For this review, take the finished solid that the model builds, in its own axes (mm). A direction names the side the tool comes from. Give positions to 0.01 mm unless a question says otherwise; leave off trailing zeros. Write each loop counter-clockwise with the first axis right and the second up, starting at its lowest first coordinate (ties: lowest second). Pieces come first, ordered by that corner, then holes. Notation, with made-up numbers: M 77,-4 L 135,-4 A27 cw 135,26 Z; hole C 47,-28.5 d7. An arc over 180 degrees is marked long. One line per item, written item: value. Start each with the question number.
Item 1: To check wall thickness, follow probe 1 along X at (y, z) = (-0.9, 15); probe 2 along X at (y, z) = (2.5, 4); probe 3 along X at (y, z) = (-1.5, 21.25). State the ranges of each line that lie inside material, in increasing order.
Item 2: Consider section D-D, the plane z = 15. Write out the cut boundary in (x, y), and give its area (3 significant figures).
Item 3: Tool access review of faces 1 (the face through (31.879, 2.186, 14.79)), 2 (the face through (38.4, 1.2, 14.8)): name each direction out of +Z, -Z, +X, -X, +Y, -Y from which nothing blocks a thin tool from reaching the whole face with its end or side.
Item 4: Consider section B-B, the plane x = 0. Write out the cut boundary in (y, z).
Item 5: Clearance check with flat-ended pins moving along their axes: pin 1 Ø1.2 at (y, z) = (-1, 17.5) entering from -X; pin 2 Ø1.2 at (y, z) = (-1.5, 11.5) entering from +X; pin 3 Ø9 at (x, z) = (13, 17.5) entering from +Y. State where each tip first meets the part, or that it passes through.
Item 6: Consider section A-A, the plane z = 12. Write out the cut boundary in (x, y), and give its area (3 significant figures).
Item 7: Mouldability with a two-part tool opening along X and no side actions: class faces 3 (the face through (0, 2.071, 8)), 4 (the face through (-38.4, 1.2, 14.8)), 5 (the face through (-1, 0, 0)) as released by +X, released by -X, zero draft, split by the parting line, or undercut.
Item 8: Consider section C-C, the plane z = 5.5. Write out the cut boundary in (x, y).
```python
from build123d import *

# Parameters (mm, degrees)
BOSS_EXTRUDE1_DEPTH = 30
FILLET1_R           = 5
SKETCH2_R           = 5
CUT_EXTRUDE1_DEPTH  = 30


with BuildPart() as part:
    # Sketch1 → Boss-Extrude1 (new body)
    with BuildSketch(Plane.XY):
        Polygon((37.92, -2.070510622), (37.92, 2.070510622), (35.334085277, 2.070510622), (33.1622407, 1.057762863), (33.014324308, 1.374970589), (34.505914723, 2.070510622), (31.92, 2.070510622), (-31.92, 2.070510622), (-34.505914723, 2.070510622), (-33.014324308, 1.374970589), (-33.1622407, 1.057762863), (-35.334085277, 2.070510622), (-37.92, 2.070510622), (-37.92, -2.070510622), align=None)
        Polygon((-39.732615574, 2.915747145), (-37.92, 2.070510622), (-35.334085277, 2.070510622), (-39.270755184, 3.906209947), align=None)
        Polygon((-34.505914723, 2.070510622), (-31.92, 2.070510622), (-38.660978403, 5.213880475), (-39.122838793, 4.223417673), align=None)
        Polygon((31.92, 2.070510622), (34.505914723, 2.070510622), (39.122838793, 4.223417673), (38.660978403, 5.213880475), align=None)
        Polygon((35.334085277, 2.070510622), (37.92, 2.070510622), (39.732615574, 2.915747145), (39.270755184, 3.906209947), align=None)
    extrude(amount=BOSS_EXTRUDE1_DEPTH)

    # Fillet1
    # the kernel refuses this fillet: 5 mm, written as the material it adds along each edge
    with BuildSketch(Plane(origin=(37.92, 2.070510622, 0), x_dir=(0, -1, 0), z_dir=(0, 0, 1))) as fillet1_piece_1:
        with BuildLine():
            CenterArc((3.007110881, 5), FILLET1_R, 219.603933445, 50.396066555)
            Line((-0.845236523, 1.812615574), (-0.922283472, 1.748867886))
            ThreePointArc((-0.922283472, 1.748867886), (-0.51324904, 0.864045961), (-0.090630779, -0.042261826))
            Line((-0.090630779, -0.042261826), (0, -0.1))
            Line((0, -0.1), (3.007110881, -0.1))
            Line((3.007110881, -0.1), (3.007110881, 0))
        make_face()
    extrude(amount=30)
    with BuildSketch(Plane(origin=(-37.92, 2.070510622, 0), x_dir=(0, -1, 0), z_dir=(0, 0, 1))) as fillet1_piece_2:
        with BuildLine():
            CenterArc((3.007110881, -5), FILLET1_R, 90, 50.396066555)
            Line((-0.845236523, -1.812615574), (-0.922283472, -1.748867886))
            ThreePointArc((-0.922283472, -1.748867886), (-0.51324904, -0.864045961), (-0.090630779, 0.042261826))
            Line((-0.090630779, 0.042261826), (0, 0.1))
            Line((0, 0.1), (3.007110881, 0.1))
            Line((3.007110881, 0.1), (3.007110881, 0))
        make_face()
    extrude(amount=30)
    with BuildSketch(Plane(origin=(31.92, 2.070510622, 0), x_dir=(-1, 0, 0), z_dir=(0, 0, 1)), Plane(origin=(-31.92, 2.070510622, 0), x_dir=(-0.9063077870366495, 0.4226182617407004, 0), z_dir=(0, 0, 1))) as fillet1_piece_3:
        with BuildLine():
            CenterArc((FILLET1_R * 0.221694662643, -FILLET1_R), FILLET1_R, 90, 25)
            Line((-FILLET1_R * 0.200923599098, -FILLET1_R * 0.0936922129634), (-FILLET1_R * 0.209375964333, -FILLET1_R * 0.0755660572226))
            Line((-FILLET1_R * 0.209375964333, -FILLET1_R * 0.0755660572226), (-FILLET1_R * 0.00443389325286, FILLET1_R * 0.02))
            Line((-FILLET1_R * 0.00443389325286, FILLET1_R * 0.02), (FILLET1_R * 0.221694662643, FILLET1_R * 0.02))
            Line((FILLET1_R * 0.221694662643, FILLET1_R * 0.02), (FILLET1_R * 0.221694662643, 0))
        make_face()
    extrude(amount=30)

    # Sketch2 → Cut-Extrude1 (cut)
    with BuildSketch(Plane(origin=(0, 2.070510622, 0), x_dir=(1, 0, 0), z_dir=(0, 1, 0))):
        with Locations(Location((0, -15, 0), (0, 0, 270))):
            Circle(SKETCH2_R)
    extrude(amount=-CUT_EXTRUDE1_DEPTH, mode=Mode.SUBTRACT)


solid = part.part
```
Model answer:
1. probe 1: x = -37.92 to -5, 5 to 37.92
1. probe 2: x = -39.29 to -36.26, -35.43 to -32.84, 32.84 to 35.43, 36.26 to 39.29
1. probe 3: x = -37.92 to 37.92
2. outline: M -39.73,2.92 A5 cw -37.92,-0.94 L -37.92,-2.07 L -5,-2.07 L -5,2.07 L -30.81,2.07 A5 cw -32.92,2.54 L -38.66,5.21 L -39.12,4.22 L -33.01,1.37 L -33.16,1.06 L -39.27,3.91 Z; M 5,-2.07 L 37.92,-2.07 L 37.92,-0.94 A5 cw 39.73,2.92 L 39.27,3.91 L 33.16,1.06 L 33.01,1.37 L 39.12,4.22 L 38.66,5.21 L 32.92,2.54 A5 cw 30.81,2.07 L 5,2.07 Z
2. area: 295 mm2
3. face 1: +Z, -Z, +Y
3. face 2: +Z, -Z, +X, -Y
4. outline: M -2.07,0 L 2.07,0 L 2.07,10 L -2.07,10 Z; M -2.07,20 L 2.07,20 L 2.07,30 L -2.07,30 Z
5. pin 1: stops at x = -37.95
5. pin 2: stops at x = 37.92
5. pin 3: stops at y = 2.07
6. outline: M -39.73,2.92 A5 cw -37.92,-0.94 L -37.92,-2.07 L -4,-2.07 L -4,2.07 L -30.81,2.07 A5 cw -32.92,2.54 L -38.66,5.21 L -39.12,4.22 L -33.01,1.37 L -33.16,1.06 L -39.27,3.91 Z; M 4,-2.07 L 37.92,-2.07 L 37.92,-0.94 A5 cw 39.73,2.92 L 39.27,3.91 L 33.16,1.06 L 33.01,1.37 L 39.12,4.22 L 38.66,5.21 L 32.92,2.54 A5 cw 30.81,2.07 L 4,2.07 Z
6. area: 303 mm2
7. face 3: undercut
7. face 4: released by -X
7. face 5: zero draft
8. outline: M -39.73,2.92 A5 cw -37.92,-0.94 L -37.92,-2.07 L 37.92,-2.07 L 37.92,-0.94 A5 cw 39.73,2.92 L 39.27,3.91 L 33.16,1.06 L 33.01,1.37 L 39.12,4.22 L 38.66,5.21 L 32.92,2.54 A5 cw 30.81,2.07 L -30.81,2.07 A5 cw -32.92,2.54 L -38.66,5.21 L -39.12,4.22 L -33.01,1.37 L -33.16,1.06 L -39.27,3.91 Z
